CAD build for the part. Positions are in the model's coordinates, mm. A direction names the side the tool comes from. Coordinates: 2 decimals unless noted, no trailing zeros. Loops run counter-clockwise (first coordinate to the right, second up) from the corner with the lowest first, then second, coordinate; pieces in that order, holes last. Notation, with made-up numbers: (41.25, 77) -> (45.25, 77) arc R22 ccw to (45.25, 99) -> close; hole circle Ø3 at (-9.75, 11). An arc over 180 degrees is marked (long way). Write each question's results on one line, items separated by ' | '.
```python
from build123d import *

# Parameters (mm, degrees)
SKETCH_1_W      = 150
SKETCH_1_H      = 80
EXTRUDE_1_DEPTH = 10
MM_1_D          = 11
MM_1_DEPTH      = 24.5
MM_1_TIP        = 3.304733405


with BuildPart() as part:
    # 草图1 → 凸台-拉伸1 (new body)
    with BuildSketch(Plane.XY):
        Rectangle(SKETCH_1_W, SKETCH_1_H)
        with BuildLine():
            Line((-55.5, -20), (-55.5, -30))
            ThreePointArc((-55.5, -30), (-60, -34.5), (-64.5, -30))
            Line((-64.5, -30), (-64.5, -20))
            ThreePointArc((-64.5, -20), (-60, -15.5), (-55.5, -20))
        make_face(mode=Mode.SUBTRACT)
        with BuildLine():
            Line((-55.5, 20), (-55.5, 30))
            ThreePointArc((-55.5, 30), (-60, 34.5), (-64.5, 30))
            Line((-64.5, 30), (-64.5, 20))
            ThreePointArc((-64.5, 20), (-60, 15.5), (-55.5, 20))
        make_face(mode=Mode.SUBTRACT)
        with BuildLine():
            Line((55.5, -20), (55.5, -30))
            ThreePointArc((55.5, -30), (60, -34.5), (64.5, -30))
            Line((64.5, -30), (64.5, -20))
            ThreePointArc((64.5, -20), (60, -15.5), (55.5, -20))
        make_face(mode=Mode.SUBTRACT)
        with BuildLine():
            Line((55.5, 20), (55.5, 30))
            ThreePointArc((55.5, 30), (60, 34.5), (64.5, 30))
            Line((64.5, 30), (64.5, 20))
            ThreePointArc((64.5, 20), (60, 15.5), (55.5, 20))
        make_face(mode=Mode.SUBTRACT)
    extrude(amount=EXTRUDE_1_DEPTH)

    # 大小mm 暗销孔1
    with Locations(Plane(origin=(0, 0, 0), x_dir=(-1, 0, 0), z_dir=(0, 0, -1))):
        with Locations((0, 0)):
            Hole(MM_1_D / 2, depth=MM_1_DEPTH)
            with Locations((0, 0, -(MM_1_DEPTH + MM_1_TIP / 2))):  # 118° drill point
                Cone(0, MM_1_D / 2, MM_1_TIP, mode=Mode.SUBTRACT)


solid = part.part
```
Q1. Pull direction X, two halves, no side cores. Call faces 1 (the flat face through (-1, 9, 10)), 2 (the flat face through (-75, -1, 5)), 3 (the cylindrical face through (-60.1, 15.5, 4.9)): +X half, -X half, draft (parallel to the pull), parting line (faces both ways), or undercut.
Results are:
face 1: draft | face 2: -X half | face 3: undercut
Q2. Wall check: L1, parallel to X at y = -20.5, z = 0.5; L2, parallel to X at y = 16.5, z = 1.5; L3, parallel to Y at x = -62.5, z = 7. Give the ranges that are in metal, low to high. Write a range as from..to.
Results are:
L1: -75..-64.5, -55.5..55.5, 64.5..75 | L2: -75..-62.83, -57.17..57.17, 62.83..75 | L3: -40..-33.74, -16.26..16.26, 33.74..40
Q3. Cut at A-A on y = 0. Write the cut outline in (x, z), and give its area (3 significant figures).
Results are:
outline: (-75, 0) -> (-5.5, 0) -> (-5.5, 10) -> (-75, 10) -> close; (5.5, 0) -> (75, 0) -> (75, 10) -> (5.5, 10) -> close | area: 1,390 mm^2
Q4. Drop a flat-ended pin along its axis: pin 1 (3 mm diameter, centred on x = 49, y = -19, fed in from -Z). Give the stop position or say it passes through.
Results are:
pin 1: z = 0
Q5. Cut at D-D on z = 8. Write the cut outline in (x, y).
Results are:
outline: (-75, -40) -> (75, -40) -> (75, 40) -> (-75, 40) -> close; hole (-64.5, -30) arc R4.5 ccw to (-55.5, -30) -> (-55.5, -20) arc R4.5 ccw to (-64.5, -20) -> close; hole (-64.5, 20) arc R4.5 ccw to (-55.5, 20) -> (-55.5, 30) arc R4.5 ccw to (-64.5, 30) -> close; hole circle Ø11 at (0, 0); hole (55.5, -30) arc R4.5 ccw to (64.5, -30) -> (64.5, -20) arc R4.5 ccw to (55.5, -20) -> close; hole (55.5, 20) arc R4.5 ccw to (64.5, 20) -> (64.5, 30) arc R4.5 ccw to (55.5, 30) -> close
Q6. Cut at B-B on x = -60. Write the cut outline in (y, z).
Results are:
outline: (-40, 0) -> (-34.5, 0) -> (-34.5, 10) -> (-40, 10) -> close; (-15.5, 0) -> (15.5, 0) -> (15.5, 10) -> (-15.5, 10) -> close; (34.5, 0) -> (40, 0) -> (40, 10) -> (34.5, 10) -> close
Q7. Cut at C-C on x = 0. Write the cut outline in (y, z), and give its area (3 significant figures).
Results are:
outline: (-40, 0) -> (-5.5, 0) -> (-5.5, 10) -> (-40, 10) -> close; (5.5, 0) -> (40, 0) -> (40, 10) -> (5.5, 10) -> close | area: 690 mm^2
Q8. Which spindle directions (+Z, -Z, +X, -X, +Y, -Y) get a long thin tool onto all of the face, cutting with end or side? Do faces 4 (the flat face through (-1, 9, 0)), 5 (the flat face through (64.5, 25, 5)). Say none if no direction does.
Results are:
face 4: -Z, +X, -X, +Y, -Y | face 5: +Z, -Z
